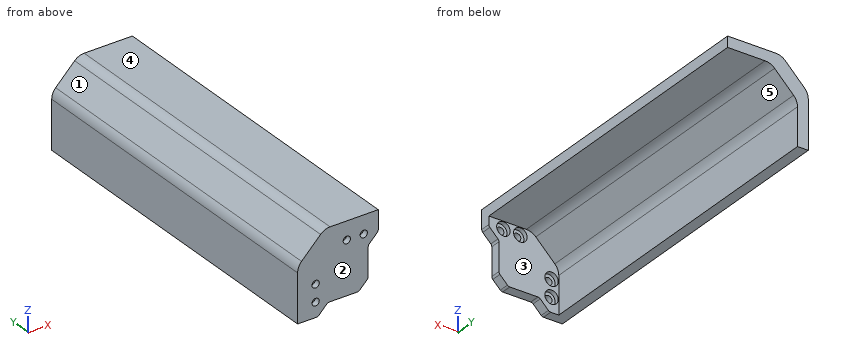
from build123d import *

# Parameters (mm, degrees)
BOSS_EXTRUDE1_DEPTH                                  = 7.5
FILLET1_R                                            = 2.5
BOSS_EXTRUDE2_DEPTH                                  = 250
CHAMFER1_SIZE                                        = 20
FILLET2_R                                            = 10
SKETCH3_R                                            = 2.7
CUT_EXTRUDE1_DEPTH                                   = 265.007575649
REFRENTADO_PARA_TORNILLO_CON_CABEZA_PLAN_D           = 5.3
REFRENTADO_PARA_TORNILLO_CON_CABEZA_PLAN_CBORE_D     = 10
REFRENTADO_PARA_TORNILLO_CON_CABEZA_PLAN_CBORE_DEPTH = 3.3


with BuildPart() as part:
    # Sketch1 → Boss-Extrude1 (new body)
    with BuildSketch(Plane(origin=(0, 0, 0), x_dir=(1, 0, 0), z_dir=(0, 1, 0))):
        Polygon((0, 0), (0, 60), (15, 60), (22.5, 52.5), (45.428932188, 52.5), (52.5, 45.428932188), (52.5, 22.5), (60, 15), (60, 0), align=None)
    extrude(amount=BOSS_EXTRUDE1_DEPTH)

    # Fillet1
    fillet1_edges = [part.edges().sort_by_distance(p)[0] for p in [
        (15, 3.75, -60),
        (22.5, 3.75, -52.5),
        (45.428932188, 3.75, -52.5),
        (52.5, 3.75, -45.428932188),
        (52.5, 3.75, -22.5),
        (60, 3.75, -15),
    ]]
    fillet(fillet1_edges, radius=FILLET1_R)

    # Sketch2 → Boss-Extrude2 (add)
    with BuildSketch(Plane(origin=(0, 7.5, 0), x_dir=(1, 0, 0), z_dir=(0, 1, 0))):
        Polygon((0, 60), (0, 0), (60, 0), (60, 8), (8, 8), (8, 60), align=None)
    extrude(amount=BOSS_EXTRUDE2_DEPTH)

    # Chamfer1
    chamfer1_edges = [part.edges().sort_by_distance(p)[0] for p in [
        (0, 128.75, 0),
        (8, 132.5, -8),
    ]]
    chamfer(chamfer1_edges, length=CHAMFER1_SIZE)

    # Fillet2
    fillet2_edges = [part.edges().sort_by_distance(p)[0] for p in [
        (20, 128.75, 0),
        (0, 128.75, -20),
        (8, 132.5, -28),
        (28, 132.5, -8),
    ]]
    fillet(fillet2_edges, radius=FILLET2_R)

    # Sketch3 → Cut-Extrude1 (cut, through all)
    with BuildSketch(Plane(origin=(0, 7.5, 0), x_dir=(1, 0, 0), z_dir=(0, 1, 0))):
        with Locations(Location((36.6, 13.4, 0), (0, 0, 270))):
            Circle(SKETCH3_R)
        with Locations(Location((49.187905991, 13.4, 0), (0, 0, 270))):
            Circle(SKETCH3_R)
        with Locations(Location((13.4, 49.187905991, 0), (0, 0, 90))):
            Circle(SKETCH3_R)
        with Locations(Location((13.4, 36.6, 0), (0, 0, 90))):
            Circle(SKETCH3_R)
    extrude(amount=-CUT_EXTRUDE1_DEPTH, mode=Mode.SUBTRACT)

    # Refrentado para tornillo con cabeza plana de M51 (through all)
    with Locations(Plane(origin=(0, 7.5, 0), x_dir=(1, 0, 0), z_dir=(0, 1, 0))):
        with Locations((13.4, 49.187905991), (13.4, 36.6), (36.6, 13.4), (49.187905991, 13.4)):
            CounterBoreHole(REFRENTADO_PARA_TORNILLO_CON_CABEZA_PLAN_D / 2, REFRENTADO_PARA_TORNILLO_CON_CABEZA_PLAN_CBORE_D / 2, REFRENTADO_PARA_TORNILLO_CON_CABEZA_PLAN_CBORE_DEPTH)


solid = part.part
Read the model definition and answer for the solid it produces. Units are mm, in the model's axes. Face numbers are marked on the shaded views. A direction names the side the tool comes from. Round coordinates to 2 decimals unless told otherwise and drop trailing zeros. Write each loop counter-clockwise with the first axis right and the second up, starting at its lowest first coordinate (ties: lowest second). Pieces come first, ordered by that corner, then holes.
Q1. A tool of negligible diameter and unlimited length cuts with its end or side. For the marked faces 4 and 5, from which of +Z, -Z, +X, -X, +Y, -Y can it reach the whole face along a straight path? Write none if from no direction.
Values:
face 4: +Z, +X, -X, +Y, -Y
face 5: -Z, +X, +Y
Q2. The mould has two halves that part along Y. Classify the marked faces 1, 2 and 3: released by +Y, released by -Y, zero draft, split by the parting line, or undercut.
Values:
face 1: zero draft
face 2: released by -Y
face 3: released by +Y
Q3. Straight lines are drawn through the part: line 1 (X direction, y = 2.6, z = -36.6); line 2 (Z direction, x = 13.4, y = 1.6); line 3 (Z direction, x = 36.6, y = 5.95). For each, find the intervals that lie inside material, in ascending order.
Values:
line 1: x = 0 to 10.7, 16.1 to 52.5
line 2: z = -60 to -51.89, -46.49 to -39.3, -33.9 to -6.6
line 3: z = -52.5 to -18.4, -8.4 to 0
Q4. Find section C-C on y = 173.5. Determine the outline of the cut face in (x, z), and give its area (3 significant figures).
Values:
outline: (0, -60) - (8, -60) - (8, -32.14) arc R10 cw to (10.93, -25.07) - (25.07, -10.93) arc R10 cw to (32.14, -8) - (60, -8) - (60, 0) - (24.14, 0) arc R10 ccw to (17.07, -2.93) - (2.93, -17.07) arc R10 ccw to (0, -24.14) - close
area: 896 mm2
Q5. Find section B-B on x = 36.6. Determine the outline of the cut face in (y, z).
Values:
outline: (0, -52.5) - (7.5, -52.5) - (7.5, -18.4) - (4.2, -18.4) - (4.2, -16.1) - (0, -16.1) - close; (0, -10.7) - (4.2, -10.7) - (4.2, -8.4) - (7.5, -8.4) - (7.5, -8) - (257.5, -8) - (257.5, 0) - (0, 0) - close
Q6. Flat-ended cylindrical pins translate along their axes: P1, Ø8, axis at x = 38.5, y = 4, coming from the -Z side; P2, Ø10, axis at x = 29, z = -53, coming from the +Y side; P3, Ø22.5, axis at x = 51, y = 185, coming from the -Z side. Find the tip coordinate at first contact, or state that the pin passes through.
Values:
P1: stops at z = -52.5
P2: stops at y = 7.5
P3: stops at z = -8
Q7. Find section A-A on z = -36.6. Determine the outline of the cut face in (x, y).
Values:
outline: (0, 0) - (10.7, 0) - (10.7, 4.2) - (8.4, 4.2) - (8.4, 7.5) - (8, 7.5) - (8, 257.5) - (0, 257.5) - close; (16.1, 0) - (52.5, 0) - (52.5, 7.5) - (18.4, 7.5) - (18.4, 4.2) - (16.1, 4.2) - close
